from build123d import *

# Parameters (mm, degrees)
SKETCH1_R               = 1.25
BOSS_EXTRUDE1_DEPTH     = 11
SKETCH1_3_R             = 1.25
BOSS_EXTRUDE2_DEPTH     = 5
CHAMFER1_SIZE           = 0.5
M2_5_TAPPED_HOLE1_D     = 2.05
M2_5_TAPPED_HOLE1_DEPTH = 10
M2_5_TAPPED_HOLE1_TIP   = 0.615882135


with BuildPart() as part:
    # Sketch1 → Boss-Extrude1 (new body)
    # profile 1 of 2: a face of its own
    with BuildSketch(Plane(origin=(0, 0, 0), x_dir=(1, 0, 0), z_dir=(0, 1, 0))):
        Polygon((-2.309401077, 0), (-1.154700538, -2), (1.154700538, -2), (2.309401077, 0), (1.154700538, 2), (-1.154700538, 2), align=None)
        Circle(SKETCH1_R, mode=Mode.SUBTRACT)
    # profile 2 of 2: a face of its own
    with BuildSketch(Plane(origin=(0, 0, 0), x_dir=(1, 0, 0), z_dir=(0, 1, 0))):
        Circle(SKETCH1_R)
    extrude(amount=BOSS_EXTRUDE1_DEPTH)

    # Sketch1_3 → Boss-Extrude2 (add)
    with BuildSketch(Plane(origin=(0, 0, 0), x_dir=(1, 0, 0), z_dir=(0, 1, 0))):
        with Locations(Location((0, 0, 0), (0, 0, 270))):
            Circle(SKETCH1_3_R)
    extrude(amount=-BOSS_EXTRUDE2_DEPTH)

    # Chamfer1
    chamfer1_edges = [part.edges().sort_by_distance(p)[0] for p in [
        (0, -5, -1.25),
    ]]
    chamfer(chamfer1_edges, length=CHAMFER1_SIZE)

    # M2.5 Tapped Hole1
    with Locations(Plane(origin=(0, 11, 0), x_dir=(1, 0, 0), z_dir=(0, 1, 0))):
        with Locations((0, 0)):
            Hole(M2_5_TAPPED_HOLE1_D / 2, depth=M2_5_TAPPED_HOLE1_DEPTH)
            with Locations((0, 0, -(M2_5_TAPPED_HOLE1_DEPTH + M2_5_TAPPED_HOLE1_TIP / 2))):  # 118° drill point
                Cone(0, M2_5_TAPPED_HOLE1_D / 2, M2_5_TAPPED_HOLE1_TIP, mode=Mode.SUBTRACT)


solid = part.part
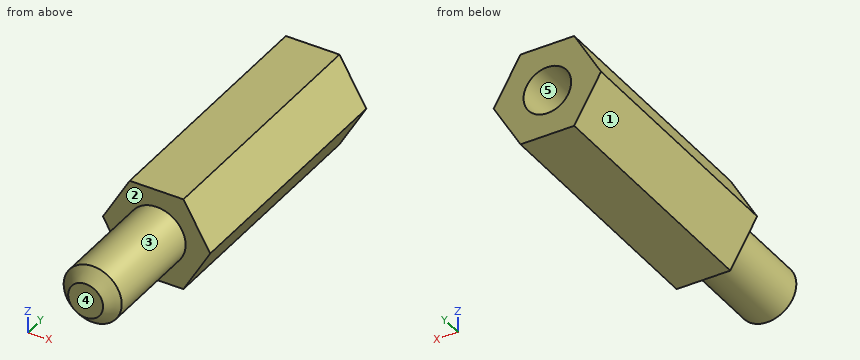
The model under review builds one solid part; all positions refer to its coordinate system, in mm. Face numbers are marked on the shaded views. A direction names the side the tool comes from. Give positions to 0.01 mm unless a question says otherwise; leave off trailing zeros. Write each loop counter-clockwise with the first axis right and the second up, starting at its lowest first coordinate (ties: lowest second). Pieces come first, ordered by that corner, then holes.
1. Draft analysis for pull direction X (two halves, no side actions). For the marked faces 3, 4 and 5, state which applies: +X half, -X half, draft (parallel to the pull), parting line (faces both ways), or undercut.
2. Add section D-D, the plane y = -3.5. Write out the cut boundary in (x, z).
3. Wall thickness on L1, parallel to Z at x = 0, y = 5 (3 decimals); L2, parallel to Y at x = 1.1, z = -1; L3, parallel to X at y = 1.75, z = 0.05: over which ranges is each line inside the solid? List them lowest first.
4. Add section A-A, the plane y = 5. Write out the cut boundary in (x, z) (3 decimals).
5. Add section B-B, the plane z = 1.5. Write out the cut boundary in (x, y).
6. For P1, Ø2, axis at y = 5.5, z = 0.5, coming from the +X side; P2, Ø1, axis at y = -3, z = -0.5, coming from the -X side; P3, Ø1, axis at y = 0.5, z = 1.5, coming from the +X side, all flat-tipped, find the tip position at first contact; note any pin that passes through.
7. Add section C-C, the plane y = 0.75. Write out the cut boundary in (x, z).
8. Tool access review of the marked faces 1 and 2: name each direction out of +Z, -Z, +X, -X, +Y, -Y from which nothing blocks a thin tool from reaching the whole face with its end or side.
Worked answers:
1. face 3: parting line
1. face 4: draft
1. face 5: undercut
2. outline: circle Ø2.5 at (0, 0)
3. L1: z = -2 to -1.025, 1.025 to 2
3. L2: y = 0 to 11
3. L3: x = -2.28 to -1.02, 1.02 to 2.28
4. outline: (-2.309, 0) - (-1.155, -2) - (1.155, -2) - (2.309, 0) - (1.155, 2) - (-1.155, 2) - close; hole circle Ø2.05 at (0, 0)
5. outline: (-1.44, 0) - (1.44, 0) - (1.44, 11) - (-1.44, 11) - close
6. P1: stops at x = 2.31
6. P2: stops at x = -1.25
6. P3: stops at x = 1.73
7. outline: (-2.31, 0) - (-1.15, -2) - (1.15, -2) - (2.31, 0) - (1.15, 2) - (-1.15, 2) - close; hole circle Ø1.22 at (0, 0)
8. face 1: -Z, -X, +Y, -Y
8. face 2: -Y
